Can you work these out from the model? Positions are in its coordinate system, mm. Face numbers are marked on the shaded views. A direction names the side the tool comes from. Coordinates: 2 decimals unless noted, no trailing zeros. Order: outer loops, then holes, each group sorted by start corner. A loop starts at its lowest first (then second) coordinate and runs counter-clockwise, first axis right, second up. Notation, with made-up numbers: (21, -3) -> (77, -3) arc R9 cw to (77, 14) -> close; hole circle Ø10 at (78.25, -39.5). An arc over 180 degrees is marked (long way). Use a Markdown table: item, result. Add a question column.
1. Suppose I cut it at C-C, the plane y = 45.5. List the corners of the cut face in (x, z) for me.
2. For pin 1 Ø12 at (y, z) = (44.5, 95.5) entering from +X; pin 2 Ø5 at (x, z) = (30, 28.5) entering from +Y; pin 3 Ø3 at (x, y) = (37.5, 4) entering from +Z; pin 4 Ø3 at (x, y) = (33.5, 6) entering from -Z, each with a flat end and sliding along its axis, tell me the tip position at first contact or that it passes through.
3. Suppose I cut it at D-D, the plane z = 57. List the corners of the cut face in (x, y) for me (3 decimals), then the cut area to 3 significant figures.
4. Suppose I cut it at A-A, the plane z = 150. List the corners of the cut face in (x, y) for me (3 decimals), then the cut area to 3 significant figures.
5. Suppose I cut it at B-B, the plane x = 19.5. List the corners of the cut face in (y, z) for me, then the cut area to 3 significant figures.
6. For the marked faces 1 and 2, which set-ups out of +Z, -Z, +X, -X, +Y, -Y let a thin tool reach every point of the face, with its end or its side?
7. If I drill on line 1 along Y through (x, z) = (15, 10); line 2 along Z through (x, y) = (32, 5), over which ranges is the centre line in solid material (lowest first)? Write a range as from..to.
Autodesk Inventor part; units mm, degrees
ref_plane "YZ Plane" through (0, 0, 0) normal (1, 0, 0) x (0, 1, 0)
ref_plane "XZ Plane" through (0, 0, 0) normal (0, 1, 0) x (-1, 0, 0)
ref_plane "XY Plane" through (0, 0, 0) normal (0, 0, 1) x (1, 0, 0)
sketch "Sketch1" plane through (0, 0, 0) normal (0, 0, 1) x (1, 0, 0)
  line L0 (0, 0) -> (6.35, 0)
  line L1 (6.35, 0) -> (6.35, 50.8)
  line L2 (6.35, 50.8) -> (0, 50.8)
  line L3 (0, 50.8) -> (0, 0)
  line L4 (0, 0) -> (50.8, 0)
  line L5 (50.8, 0) -> (50.8, 6.35)
  line L6 (50.8, 6.35) -> (0, 6.35)
  line L7 (0, 6.35) -> (0, 0)
  dimension "d0" = 6.35
  dimension "d1" = 50.8
  dimension "d2" = 50.8
  dimension "d3" = 6.35
extrude "Extrusion1" add sketch "Sketch1" along normal blind 165.1
fillet "Fillet1" radius 3.175 3 edges at (6.35, 50.8, 82.55) (6.35, 6.35, 82.55) (50.8, 6.35, 82.55)
sketch "Sketch2" plane through (0, 0, 0) normal (0, -1, 0) x (1, 0, 0)
  line L0 (0, 165.1) -> (50.8, 165.1)
  line L1 (0, 0) -> (0, 165.1)
  line L2 (0, 0) -> (50.8, 0)
  line L3 (50.8, 0) -> (50.8, 165.1)
  line L4 (50.8, 165.1) -> (50.8, 0)
  line L5 (6.35, 165.1) -> (50.8, 165.1)
  line L6 (50.8, 165.1) -> (50.8, 120.65)
  line L7 (50.8, 120.65) -> (6.35, 120.65)
  line L8 (6.35, 120.65) -> (6.35, 165.1)
  dimension "d7" = 44.45
extrude "Extrusion2" cut sketch "Sketch2" against normal blind 165.1 contours L0 L3 L7 L8
sketch "Sketch3" plane through (0, 0, 0) normal (-1, 0, 0) x (0, 0, 1)
  circle A0 centre (135.255, 4.445) radius 2.54
  circle A1 centre (154.305, 4.445) radius 2.54
  circle A2 centre (154.305, 41.275) radius 2.54
  circle A3 centre (135.255, 41.275) radius 2.54
  line L0 (124.46, 45.72) -> (124.46, 0)
  line L1 (144.78, 45.72) -> (124.46, 45.72)
  line L2 (165.1, 45.72) -> (144.78, 45.72)
  line L3 (165.1, 0) -> (165.1, 45.72)
  line L4 (124.46, 0) -> (165.1, 0)
  point P0 (0, 0)
extrude "Extrusion3" cut sketch "Sketch3" against normal blind 165.1 contours A0 | A1 | A2 | A3
properties part number "lbeam final"
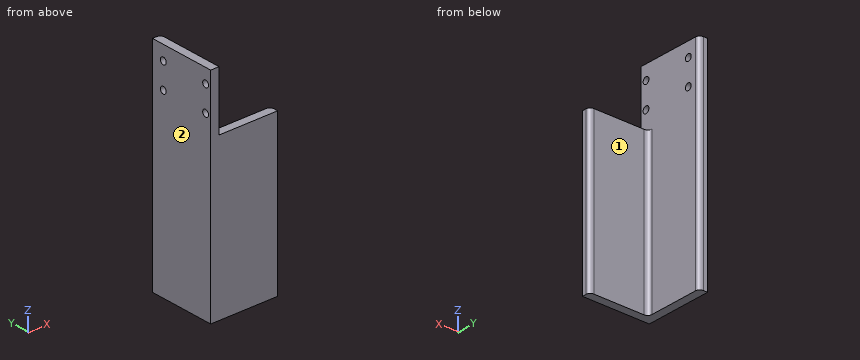
Worked out:
| question | item | result |
|---|---|---|
| 1 | outline | (0, 0) -> (6.35, 0) -> (6.35, 165.1) -> (0, 165.1) -> close |
| 2 | pin 1 | stops at x = 6.35 |
| 2 | pin 2 | stops at y = 6.35 |
| 2 | pin 3 | stops at z = 120.65 |
| 2 | pin 4 | stops at z = 0 |
| 3 | outline | (0, 0) -> (50.8, 0) -> (50.8, 3.175) arc R3.175 ccw to (47.625, 6.35) -> (9.525, 6.35) arc R3.175 cw to (6.35, 9.525) -> (6.35, 47.625) arc R3.175 ccw to (3.175, 50.8) -> (0, 50.8) -> close |
| 3 | area | 603 mm² |
| 4 | outline | (0, 0) -> (6.35, 0) -> (6.35, 47.625) arc R3.175 ccw to (3.175, 50.8) -> (0, 50.8) -> close |
| 4 | area | 320 mm² |
| 5 | outline | (0, 0) -> (6.35, 0) -> (6.35, 120.65) -> (0, 120.65) -> close |
| 5 | area | 766 mm² |
| 6 | face 1 | +Z, -Z, +X, +Y |
| 6 | face 2 | +Z, -Z, -X, +Y, -Y |
| 7 | line 1 | y = 0..6.35 |
| 7 | line 2 | z = 0..120.65 |
